Source: CAD feature listing. Evaluate the final solid. Frame: model axes, mm. Coordinates: 2 decimals unless noted, no trailing zeros. Write each loop counter-clockwise with the first axis right and the second up, starting at its lowest first coordinate (ties: lowest second). Pieces come first, ordered by that corner, then holes. Notation, with made-up numbers: (87.25, -21) -> (95.25, -21) arc R15 cw to (95.25, -12) -> close; hole circle Ø9 at (82, -21). An arc over 180 degrees is marked (long way). Write item = value, one per line.
from build123d import *

# Parameters (mm, degrees)
SKETCH1_R           = 2
SKETCH1_R_2         = 2.5
SKETCH1_R_3         = 1.5
SKETCH1_R_4         = 10
BOSS_EXTRUDE1_DEPTH = 3
FILLET1_R           = 3


with BuildPart() as part:
    # Sketch1 → Boss-Extrude1 (new body)
    with BuildSketch(Plane.XY):
        with BuildLine():
            Line((-50, -26), (-50, -36))
            Line((-50, -36), (-2.200488998, -50.66992665))
            ThreePointArc((-2.200488998, -50.66992665), (0, -51), (2.200488998, -50.66992665))
            Line((2.200488998, -50.66992665), (50, -36))
            Line((50, -36), (50, -26))
            Line((50, -26), (16.964082686, 14.00785132))
            ThreePointArc((16.964082686, 14.00785132), (0, 22), (-16.964082686, 14.00785132))
            Line((-16.964082686, 14.00785132), (-50, -26))
        make_face()
        with Locations((-25, -31)):
            Circle(SKETCH1_R, mode=Mode.SUBTRACT)
        with Locations((0, -31)):
            Circle(SKETCH1_R, mode=Mode.SUBTRACT)
        with Locations((25, -31)):
            Circle(SKETCH1_R, mode=Mode.SUBTRACT)
        with Locations((0, -43.5)):
            Circle(SKETCH1_R_2, mode=Mode.SUBTRACT)
        with Locations((14.5, 0)):
            Circle(SKETCH1_R_3, mode=Mode.SUBTRACT)
        Circle(SKETCH1_R_4, mode=Mode.SUBTRACT)
        with Locations((-14.5, 0)):
            Circle(SKETCH1_R_3, mode=Mode.SUBTRACT)
    extrude(amount=BOSS_EXTRUDE1_DEPTH)

    # Fillet1
    fillet1_edges = [part.edges().sort_by_distance(p)[0] for p in [
        (-50, -36, 1.5),
        (-50, -26, 1.5),
        (50, -26, 1.5),
        (50, -36, 1.5),
    ]]
    fillet(fillet1_edges, radius=FILLET1_R)


solid = part.part
1) Cut plane A-A, the plane y = -31. Output: boundary loops of the cut face in (x, z), and give its area (3 significant figures).
Answer block:
outline = (-50, 0) -> (-27, 0) -> (-27, 3) -> (-50, 3) -> close; (-23, 0) -> (-2, 0) -> (-2, 3) -> (-23, 3) -> close; (2, 0) -> (23, 0) -> (23, 3) -> (2, 3) -> close; (27, 0) -> (50, 0) -> (50, 3) -> (27, 3) -> close
area = 264 mm2
2) Cut plane D-D, the plane y = -43.5. Output: boundary loops of the cut face in (x, z).
Answer block:
outline = (-25.56, 0) -> (-2.5, 0) -> (-2.5, 3) -> (-25.56, 3) -> close; (2.5, 0) -> (25.56, 0) -> (25.56, 3) -> (2.5, 3) -> close
3) Material intervals for probe 1 along Y at (x, z) = (0, 1.5); probe 2 along X at (y, z) = (-30, 1.95); probe 3 along Y at (x, z) = (-25, 1.35), sorted ascending. Write a range as [from, to].
Answer block:
probe_1 = [-51, -46], [-41, -33], [-29, -10], [10, 22]
probe_2 = [-50, -26.73], [-23.27, -1.73], [1.73, 23.27], [26.73, 50]
probe_3 = [-43.67, -33], [-29, 4.28]
4) Cut plane C-C, the plane z = 2.5. Output: boundary loops of the cut face in (x, y).
Answer block:
outline = (-50, -33.78) arc R3 ccw to (-47.88, -36.65) -> (-2.2, -50.67) arc R7.5 ccw to (2.2, -50.67) -> (47.88, -36.65) arc R3 ccw to (50, -33.78) -> (50, -27.08) arc R3 ccw to (49.31, -25.17) -> (16.96, 14.01) arc R22 ccw to (-16.96, 14.01) -> (-49.31, -25.17) arc R3 ccw to (-50, -27.08) -> close; hole circle Ø4 at (-25, -31); hole circle Ø3 at (-14.5, 0); hole circle Ø20 at (0, 0); hole circle Ø5 at (0, -43.5); hole circle Ø4 at (0, -31); hole circle Ø3 at (14.5, 0); hole circle Ø4 at (25, -31)
5) Pull-direction query (X, two-part tool) for faces 1 (the cylindrical face through (-0.54, -45.94, 1.48)), 2 (the cylindrical face through (0, -33, 1)), 3 (the cylindrical face through (0, 22, 1)), 4 (the cylindrical face through (-49.43, -35.54, 1.52)); classes: +X half, -X half, draft (parallel to the pull), parting line (faces both ways), or undercut.
Answer block:
face_1 = undercut
face_2 = undercut
face_3 = parting line
face_4 = -X half
6) Cut plane B-B, the plane x = 0. Output: boundary loops of the cut face in (y, z).
Answer block:
outline = (-51, 0) -> (-46, 0) -> (-46, 3) -> (-51, 3) -> close; (-41, 0) -> (-33, 0) -> (-33, 3) -> (-41, 3) -> close; (-29, 0) -> (-10, 0) -> (-10, 3) -> (-29, 3) -> close; (10, 0) -> (22, 0) -> (22, 3) -> (10, 3) -> close
